```python
from build123d import *

# Parameters (mm, degrees)
SKETCH1_W                 = 69.85
SKETCH1_H                 = 304.8
BOSS_EXTRUDE1_DEPTH       = 25.4
FILLET1_R                 = 2.54
SKETCH2_W                 = 69.85
SKETCH2_H                 = 5.08
CUT_EXTRUDE1_DEPTH        = 5.08
SKETCH3_W                 = 50.8
SKETCH3_H                 = 304.8
CUT_EXTRUDE2_DEPTH        = 9.525
CUT_EXTRUDE3_REACH        = 71.85
SKETCH4_R                 = 2.2479
F_8_32_TAPPED_HOLE1_D     = 3.4544
F_8_32_TAPPED_HOLE1_DEPTH = 10.668
F_8_32_TAPPED_HOLE1_TIP   = 1.037806461
F_8_32_TAPPED_HOLE2_D     = 3.4544
F_8_32_TAPPED_HOLE2_DEPTH = 9.525
F_8_32_TAPPED_HOLE3_D     = 3.4544
F_8_32_TAPPED_HOLE3_DEPTH = 12.7
F_8_32_TAPPED_HOLE3_TIP   = 1.037806461
SKETCH16_W                = 9.525
SKETCH16_H                = 9.525
CUT_EXTRUDE4_DEPTH        = 127


with BuildPart() as part:
    # Sketch1 → Boss-Extrude1 (new body)
    with BuildSketch(Plane(origin=(0, 0, 0), x_dir=(1, 0, 0), z_dir=(0, 1, 0))):
        with Locations((34.925, 152.4)):
            Rectangle(SKETCH1_W, SKETCH1_H)
    extrude(amount=BOSS_EXTRUDE1_DEPTH)

    # Fillet1
    fillet1_edges = [part.edges().sort_by_distance(p)[0] for p in [
        (34.925, 0, -304.8),
        (69.85, 0, -152.4),
        (34.925, 0, 0),
        (0, 0, -152.4),
        (0, 12.7, -304.8),
        (69.85, 12.7, -304.8),
        (69.85, 12.7, 0),
        (0, 12.7, 0),
    ]]
    fillet(fillet1_edges, radius=FILLET1_R)

    # Sketch2 → Cut-Extrude1 (cut)
    with BuildSketch(Plane.XZ):
        with Locations((34.925, -180.34)):
            Rectangle(SKETCH2_W, SKETCH2_H)
        with Locations((34.925, -205.74)):
            Rectangle(SKETCH2_W, SKETCH2_H)
        with Locations((34.925, -251.46)):
            Rectangle(SKETCH2_W, SKETCH2_H)
        with Locations((34.925, -276.86)):
            Rectangle(SKETCH2_W, SKETCH2_H)
    extrude(amount=-CUT_EXTRUDE1_DEPTH, mode=Mode.SUBTRACT)

    # Sketch3 → Cut-Extrude2 (cut)
    with BuildSketch(Plane(origin=(0, 25.4, 0), x_dir=(1, 0, 0), z_dir=(0, 1, 0))):
        with Locations((34.925, 152.4)):
            Rectangle(SKETCH3_W, SKETCH3_H)
    extrude(amount=-CUT_EXTRUDE2_DEPTH, mode=Mode.SUBTRACT)

    # Sketch4 → Cut-Extrude3 (cut, up to next)
    with BuildSketch(Plane.ZY, mode=Mode.PRIVATE) as cut_extrude3_sk1:
        with Locations((-203.2, 20.6375)):
            Circle(SKETCH4_R)
    cut_extrude3_tool1 = extrude(cut_extrude3_sk1.sketch, amount=-CUT_EXTRUDE3_REACH, mode=Mode.PRIVATE) & part.part
    add(cut_extrude3_tool1.solids().sort_by_distance((0, 20.6375, -203.2))[0], mode=Mode.SUBTRACT)
    # Sketch4 → Cut-Extrude3 (cut, up to next)
    with BuildSketch(Plane.ZY, mode=Mode.PRIVATE) as cut_extrude3_sk2:
        with Locations((-228.6, 20.6375)):
            Circle(SKETCH4_R)
    cut_extrude3_tool2 = extrude(cut_extrude3_sk2.sketch, amount=-CUT_EXTRUDE3_REACH, mode=Mode.PRIVATE) & part.part
    add(cut_extrude3_tool2.solids().sort_by_distance((0, 20.6375, -228.6))[0], mode=Mode.SUBTRACT)
    # Sketch4 → Cut-Extrude3 (cut, up to next)
    with BuildSketch(Plane.ZY, mode=Mode.PRIVATE) as cut_extrude3_sk3:
        with Locations((-254, 20.6375)):
            Circle(SKETCH4_R)
    cut_extrude3_tool3 = extrude(cut_extrude3_sk3.sketch, amount=-CUT_EXTRUDE3_REACH, mode=Mode.PRIVATE) & part.part
    add(cut_extrude3_tool3.solids().sort_by_distance((0, 20.6375, -254))[0], mode=Mode.SUBTRACT)

    # #8-32 Tapped Hole1
    with Locations(Plane(origin=(0, 25.4, 0), x_dir=(1, 0, 0), z_dir=(0, 1, 0))):
        with Locations((65.0875, 298.45), (4.7625, 298.45), (65.0875, 215.9), (4.7625, 215.9), (65.0875, 133.35), (4.7625, 133.35)):
            Hole(F_8_32_TAPPED_HOLE1_D / 2, depth=F_8_32_TAPPED_HOLE1_DEPTH)
            with Locations((0, 0, -(F_8_32_TAPPED_HOLE1_DEPTH + F_8_32_TAPPED_HOLE1_TIP / 2))):  # 118° drill point
                Cone(0, F_8_32_TAPPED_HOLE1_D / 2, F_8_32_TAPPED_HOLE1_TIP, mode=Mode.SUBTRACT)

    # #8-32 Tapped Hole2
    with Locations(Plane(origin=(69.85, 0, 0), x_dir=(0, 0, -1), z_dir=(1, 0, 0))):
        with Locations((203.2, 20.6375), (228.6, 20.6375), (254, 20.6375)):
            Hole(F_8_32_TAPPED_HOLE2_D / 2, depth=F_8_32_TAPPED_HOLE2_DEPTH)

    # #8-32 Tapped Hole3
    with Locations(Plane(origin=(0, 0, 0), x_dir=(-1, 0, 0), z_dir=(0, -1, 0))):
        with Locations((-12.7, 289.56), (-57.15, 289.56), (-12.7, 264.16), (-57.15, 264.16), (-12.7, 238.76), (-57.15, 238.76), (-12.7, 218.44), (-57.15, 218.44), (-12.7, 193.04), (-57.15, 193.04), (-12.7, 167.64), (-57.15, 167.64)):
            Hole(F_8_32_TAPPED_HOLE3_D / 2, depth=F_8_32_TAPPED_HOLE3_DEPTH)
            with Locations((0, 0, -(F_8_32_TAPPED_HOLE3_DEPTH + F_8_32_TAPPED_HOLE3_TIP / 2))):  # 118° drill point
                Cone(0, F_8_32_TAPPED_HOLE3_D / 2, F_8_32_TAPPED_HOLE3_TIP, mode=Mode.SUBTRACT)

    # Sketch16 → Cut-Extrude4 (cut)
    with BuildSketch(Plane.XY):
        with Locations((65.0875, 20.6375)):
            Rectangle(SKETCH16_W, SKETCH16_H)
    extrude(amount=-CUT_EXTRUDE4_DEPTH, mode=Mode.SUBTRACT)


solid = part.part
```
Source: CAD feature listing. Evaluate the final solid. Frame: model axes, mm. A direction names the side the tool comes from. Give positions to 0.01 mm unless a question says otherwise; leave off trailing zeros. Loops run counter-clockwise (first coordinate to the right, second up) from the corner with the lowest first, then second, coordinate; pieces in that order, holes last. Notation, with made-up numbers: (68.5, 80.5) -> (103.5, 80.5) arc R13 cw to (103.5, 102.5) -> close; hole circle Ø4 at (25, -35). An arc over 180 degrees is marked (long way). Use a Markdown table: item, result. Add a question column.
(1) Ray query, line 1 (X direction, y = 18, z = -215.9) (3 decimals); line 2 (X direction, y = 5, z = -264.16); line 3 (Z direction, x = 62, y = 2.25). Return the intervals inside material, ascending.
(2) Section query B-B (x = 46). Output: boundary loops of the cut face in (y, z) (3 decimals).
(3) Pull-direction query (Z, two-part tool) for faces 1 (the face through (34, 11, -304.8)), 2 (the face through (34, 5.08, -206)), 3 (the face through (34, 0, -193)); classes: +Z half, -Z half, draft (parallel to the pull), parting line (faces both ways), or undercut.
(4) Section query A-A (z = -116). Output: boundary loops of the cut face in (x, y) (3 decimals).
(5) First-contact query: pin 1 Ø1.5 at (x, z) = (44, -276.5) entering from -Y; pin 2 Ø2 at (x, z) = (12.7, -264.16) entering from +Y (3 decimals); pin 3 Ø3 at (y, z) = (17.5, -46.5) entering from +X (3 decimals). Flat tips, straight axial feed; report the tip coordinate or a pass-through.
(6) Access query for faces 4 (the face through (65, 21, -127)), 5 (the face through (34, 0, -91)), 6 (the face through (69.85, 11, -184)), 7 (the face through (9.525, 21, -150)), 8 (the face through (34, 3, -177.8)). Directions: +Z, -Z, +X, -X, +Y, -Y. A direction counts if a zero-diameter tool reaches every point of the face in a straight line with its end or side. Return the directions, or none.
Checked values:
| question | item | result |
|---|---|---|
| 1 | line 1 | 0 to 3.035, 6.49 to 9.525, 60.325 to 63.36, 66.815 to 69.85 |
| 1 | line 2 | 0 to 10.97, 14.43 to 55.42, 58.88 to 69.85 |
| 1 | line 3 | -304.78 to -279.4, -274.32 to -254, -248.92 to -208.28, -203.2 to -182.88, -177.8 to -0.02 |
| 2 | outline | (0, -302.26) arc R2.54 ccw to (2.54, -304.8) -> (15.875, -304.8) -> (15.875, 0) -> (2.54, 0) arc R2.54 ccw to (0, -2.54) -> (0, -177.8) -> (5.08, -177.8) -> (5.08, -182.88) -> (0, -182.88) -> (0, -203.2) -> (5.08, -203.2) -> (5.08, -208.28) -> (0, -208.28) -> (0, -248.92) -> (5.08, -248.92) -> (5.08, -254) -> (0, -254) -> (0, -274.32) -> (5.08, -274.32) -> (5.08, -279.4) -> (0, -279.4) -> close |
| 3 | face 1 | -Z half |
| 3 | face 2 | undercut |
| 3 | face 3 | draft |
| 4 | outline | (0, 2.54) arc R2.54 ccw to (2.54, 0) -> (67.31, 0) arc R2.54 ccw to (69.85, 2.54) -> (69.85, 15.875) -> (9.525, 15.875) -> (9.525, 25.4) -> (0, 25.4) -> close |
| 5 | pin 1 | y = 5.08 |
| 5 | pin 2 | y = 15.875 |
| 5 | pin 3 | x = 9.525 |
| 6 | face 4 | +Z, +X, +Y |
| 6 | face 5 | +Z, -Z, +X, -X, -Y |
| 6 | face 6 | +Z, -Z, +X, +Y, -Y |
| 6 | face 7 | +Z, -Z, +Y |
| 6 | face 8 | +X, -X, -Y |
